Check sheet for the modelled part. Datum: model origin and axes. Units: mm. Coordinates: 2 decimals unless noted, no trailing zeros. Write each loop counter-clockwise with the first axis right and the second up, starting at its lowest first coordinate (ties: lowest second). Pieces come first, ordered by that corner, then holes. Notation, with made-up numbers: M 42.25,-15 L 52.25,-15 A4 cw 52.25,-8 Z; hole C -15,27 d7. An arc over 180 degrees is marked long. Answer as CSV lines item,"result". Start each with the question number.
1) Go/stop test with flat-tipped pins: pin 1 Ø5.5 at (x, y) = (-52.39, -52.39) entering from -Z; pin 2 Ø10 at (x, y) = (1.5, -48) entering from -Z. Record where each tip stops, or that it passes through.
2) Material ranges on L1, parallel to X at y = 27, z = 2.75; L2, parallel to Y at x = -31.75, z = 7.75; L3, parallel to Y at x = 54, z = 6.5, recorded low to high. Write a range as [from, to].
3) Section check C-C (x = 0). Record the cut outline in (y, z) (1 decimal), and give its area (3 significant figures).
4) Section check A-A (y = -25.4). Record the cut outline in (x, z) (1 decimal), and give its area (3 significant figures).
5) Section check D-D (z = 5). State how many separate pieces and enclosed holes the cut face has, and give its area (3 significant figures).
6) Draft check along Y on faces 1 (the cylindrical face through (-51.355, 47.738, 4.696)), 2 (the cylindrical face through (-24.82, 20.09, 4.7)), 3 (the flat face through (-1, 63.5, 5)), 4 (the flat face through (-1, 1, 0)). Enter one of: +Y half, -Y half, draft (parallel to the pull), parting line (faces both ways), or undercut.
7) Section check B-B (y = 25.4). Record the cut outline in (x, z) (1 decimal).
from build123d import *

# Parameters (mm, degrees)
SKETCH1_W           = 127
SKETCH1_H           = 127
BOSS_EXTRUDE1_DEPTH = 9.525
SKETCH2_R           = 11.1125
SKETCH2_R_2         = 8.73125
CUT_EXTRUDE1_DEPTH  = 9.525
SKETCH3_R           = 4.7625
CUT_EXTRUDE2_DEPTH  = 9.525


with BuildPart() as part:
    # Sketch1 → Boss-Extrude1 (new body)
    with BuildSketch(Plane.XY):
        Rectangle(SKETCH1_W, SKETCH1_H)
    extrude(amount=BOSS_EXTRUDE1_DEPTH)

    # Sketch2 → Cut-Extrude1 (cut)
    with BuildSketch(Plane(origin=(0, 0, 0), x_dir=(-1, 0, 0), z_dir=(0, 0, -1))):
        with Locations((0, 25.4)):
            Circle(SKETCH2_R)
        with Locations((31.75, 25.4)):
            Circle(SKETCH2_R_2)
        with Locations((0, -25.4)):
            Circle(SKETCH2_R)
    extrude(amount=-CUT_EXTRUDE1_DEPTH, mode=Mode.SUBTRACT)

    # Sketch3 → Cut-Extrude2 (cut)
    with BuildSketch(Plane(origin=(0, 0, 0), x_dir=(-1, 0, 0), z_dir=(0, 0, -1))):
        with Locations((52.3875, 52.3875)):
            Circle(SKETCH3_R)
        with Locations((52.3875, -52.3875)):
            Circle(SKETCH3_R)
        with Locations((-52.3875, 52.3875)):
            Circle(SKETCH3_R)
        with Locations((-52.3875, -52.3875)):
            Circle(SKETCH3_R)
    extrude(amount=-CUT_EXTRUDE2_DEPTH, mode=Mode.SUBTRACT)


solid = part.part
Results found:
1,pin 1,"passes through"
1,pin 2,"stops at z = 0"
2,L1,"x = [-63.5, -40.33], [-23.17, -11], [11, 63.5]"
2,L2,"y = [-63.5, 16.67], [34.13, 63.5]"
2,L3,"y = [-63.5, -56.87], [-47.91, 47.91], [56.87, 63.5]"
3,outline,"M -63.5,0 L -36.5,0 L -36.5,9.5 L -63.5,9.5 Z; M -14.3,0 L 14.3,0 L 14.3,9.5 L -14.3,9.5 Z; M 36.5,0 L 63.5,0 L 63.5,9.5 L 36.5,9.5 Z"
3,area,"786 mm2"
4,outline,"M -63.5,0 L -11.1,0 L -11.1,9.5 L -63.5,9.5 Z; M 11.1,0 L 63.5,0 L 63.5,9.5 L 11.1,9.5 Z"
4,area,"998 mm2"
5,separate pieces,"1"
5,enclosed holes,"7"
5,area,"14,800 mm2"
6,face 1,"undercut"
6,face 2,"undercut"
6,face 3,"+Y half"
6,face 4,"draft"
7,outline,"M -63.5,0 L -40.5,0 L -40.5,9.5 L -63.5,9.5 Z; M -23,0 L -11.1,0 L -11.1,9.5 L -23,9.5 Z; M 11.1,0 L 63.5,0 L 63.5,9.5 L 11.1,9.5 Z"
